Geometry: final body of the model. Coordinates: model frame, mm. A direction names the side the tool comes from. Give positions to 0.01 mm unless a question says otherwise; leave off trailing zeros. Write each loop counter-clockwise with the first axis right and the second up, starting at its lowest first coordinate (ties: lowest second). Pieces come first, ordered by that corner, then holes. Notation, with made-up numbers: (76, -34.75) -> (107, -34.75) arc R35 ccw to (107, 2.25) -> close; hole circle Ø7 at (-20, 57.5). An arc over 180 degrees is marked (long way). Answer in a Markdown table with one row per item. Add a question column.
Item 1: Section query A-A on y = 0. Output: boundary loops of the cut face in (x, z), plus the area to 3 significant figures.
Item 2: Section query C-C on z = 7.25. Output: boundary loops of the cut face in (x, y), plus the area to 3 significant figures.
Item 3: Section query B-B on x = 54. Output: boundary loops of the cut face in (y, z), plus the area to 3 significant figures.
Item 4: Access query for faces 4 (the flat face through (63, -4, 4)), 5 (the flat face through (48, 0, 7)), 6 (the flat face through (-62, -9.2, 4)), 7 (the flat face through (-74, -4.5, 4)). Directions: +Z, -Z, +X, -X, +Y, -Y. A direction counts if a zero-diameter tool reaches every point of the face in a straight line with its end or side. Return the directions, or none.
Item 5: Section query D-D on x = 19.5. Output: boundary loops of the cut face in (y, z), plus the area to 3 significant figures.
Item 6: Material intervals for probe 1 along Z at (x, y) = (-32.5, -1.5); probe 2 along Y at (x, z) = (30, 5.5); probe 3 along Y at (x, z) = (24, 7.5), sorted ascending. Write a range as from..to.
Item 7: Draft query along Z for faces 1 (the flat face through (-72.25, 7, 4)), 2 (the flat face through (-1, 0, 0)), 3 (the flat face through (-1, -12.5, 4)). Return one class per face: +Z half, -Z half, draft (parallel to the pull), parting line (faces both ways), or undercut.
```python
from build123d import *

# Parameters (mm, degrees)
SKETCH_W      = 150
SKETCH_H      = 25
PAD_DEPTH     = 3
PAD001_DEPTH  = 3
SKETCH004_W   = 150
SKETCH004_H   = 25
SKETCH004_W_2 = 96
SKETCH004_H_2 = 2.9
PAD002_DEPTH  = 3


with BuildPart() as part:
    # Sketch → Pad (new body)
    with BuildSketch(Plane.XY):
        Rectangle(SKETCH_W, SKETCH_H)
    extrude(amount=PAD_DEPTH)

    # Sketch001 (on Face6 of Pad) → Pad001 (join)
    with BuildSketch(Plane.XY.offset(3)):
        Polygon((-75, 12.5), (75, 12.5), (75, 4), (50, 4), (50, 5), (-50, 5), (-50, 4), (-52.25, 4), (-52.25, 9.2), (-72.25, 9.2), (-72.25, 4.5), (-75, 4.5), align=None)
        Polygon((-75, -12.5), (75, -12.5), (75, -4), (50, -4), (50, -5), (-50, -5), (-50, -4), (-52.25, -4), (-52.25, -9.2), (-72.25, -9.2), (-72.25, -4.5), (-75, -4.5), align=None)
    extrude(amount=PAD001_DEPTH)

    # Sketch004 (on Face12 of Pad001) → Pad002 (join)
    with BuildSketch(Plane.XY.offset(6)):
        Rectangle(SKETCH004_W, SKETCH004_H)
        Rectangle(SKETCH004_W_2, SKETCH004_H_2, mode=Mode.SUBTRACT)
    extrude(amount=PAD002_DEPTH)


solid = part.part
```
Findings below:
| question | item | result |
|---|---|---|
| 1 | outline | (-75, 0) -> (75, 0) -> (75, 3) -> (-75, 3) -> close; (-75, 6) -> (-48, 6) -> (-48, 9) -> (-75, 9) -> close; (48, 6) -> (75, 6) -> (75, 9) -> (48, 9) -> close |
| 1 | area | 612 mm^2 |
| 2 | outline | (-75, -12.5) -> (75, -12.5) -> (75, 12.5) -> (-75, 12.5) -> close; hole (-48, -1.45) -> (48, -1.45) -> (48, 1.45) -> (-48, 1.45) -> close |
| 2 | area | 3,470 mm^2 |
| 3 | outline | (-12.5, 0) -> (12.5, 0) -> (12.5, 9) -> (-12.5, 9) -> close; hole (-4, 3) -> (4, 3) -> (4, 6) -> (-4, 6) -> close |
| 3 | area | 201 mm^2 |
| 4 | face 4 | +X, -X |
| 4 | face 5 | +Z |
| 4 | face 6 | none |
| 4 | face 7 | -X |
| 5 | outline | (-12.5, 0) -> (12.5, 0) -> (12.5, 9) -> (1.45, 9) -> (1.45, 6) -> (5, 6) -> (5, 3) -> (-5, 3) -> (-5, 6) -> (-1.45, 6) -> (-1.45, 9) -> (-12.5, 9) -> close |
| 5 | area | 186 mm^2 |
| 6 | probe 1 | z = 0..3, 6..9 |
| 6 | probe 2 | y = -12.5..-5, 5..12.5 |
| 6 | probe 3 | y = -12.5..-1.45, 1.45..12.5 |
| 7 | face 1 | undercut |
| 7 | face 2 | -Z half |
| 7 | face 3 | draft |
